from build123d import *

# Parameters (mm, degrees)
SKETCH1_R           = 12.7
BOSS_EXTRUDE1_DEPTH = 25.4
CHAMFER1_SIZE       = 4.92


with BuildPart() as part:
    # Sketch1 → Boss-Extrude1 (new body)
    with BuildSketch(Plane.XY):
        Circle(SKETCH1_R)
    extrude(amount=BOSS_EXTRUDE1_DEPTH)

    # Sketch2 → Revolve1 (revolve)
    with BuildSketch(Plane(origin=(0, 0, 0), x_dir=(1, 0, 0), z_dir=(0, 1, 0))):
        with BuildLine():
            Line((0, 0), (0, 91.44))
            add(Edge.make_bspline(
                [(0, 91.44), (-22.313297432, 89.869472139), (-44.030480488, 54.776848914), (-11.128878032, 19.035751287), (-12.7, 0)],
                knots=[0, 0, 0, 0, 0.356051471, 1, 1, 1, 1], degree=3))
            Line((-12.7, 0), (0, 0))
        make_face()
    revolve(axis=Axis((0, 0, 0), (0, 0, -1)))

    # Chamfer1
    chamfer1_edges = [part.edges().sort_by_distance(p)[0] for p in [
        (-12.7, 0, 25.4),
    ]]
    chamfer(chamfer1_edges, length=CHAMFER1_SIZE)


solid = part.part
Can you work these out from the model? Positions are in its coordinate system, mm. A direction names the side the tool comes from. Give positions to 0.01 mm unless a question says otherwise; leave off trailing zeros. Loops run counter-clockwise (first coordinate to the right, second up) from the corner with the lowest first, then second, coordinate; pieces in that order, holes last. Notation, with made-up numbers: (45.25, -32) - (77.25, -32) arc R19 cw to (77.25, -20) - close; hole circle Ø6 at (10.5, -14). An arc over 180 degrees is marked (long way). One line per item, written item: value.
(1) I'm going to push flat-ended pins straight in: pin 1 (10 mm diameter, centred on x = 13.5, z = 13.5, fed in from -Y); pin 2 (5 mm diameter, centred on x = -7, y = -3.5, fed in from -Z); pin 3 (1 mm diameter, centred on x = -19, y = 12.5, fed in from +Z). Where does each tip first touch, or does it pass through?
Verdict:
pin 1: y = -9.44
pin 2: z = -90.82
pin 3: z = -32.14
(2) On a 3-axis mill with a long thin cutter (end or side, diameter ignored), from which of +Z, -Z, +X, -X, +Y, -Y can I reach the whole of each face in a straight line? I mean faces 1 (the face through (0, 0, 25.4)), 2 (the face through (-2.75, -12.4, 10.1)). Say none if no direction works.
Verdict:
face 1: +Z, +X, -X, +Y, -Y
face 2: +Z
(3) If we section it at A-A, the plane z = 15.5: List the corners of the cut face in (x, y) for me, plus the area to 3 significant figures.
Verdict:
outline: circle Ø25.4 at (0, 0)
area: 507 mm^2
